Read the model definition and answer for the solid it produces. Units are mm, in the model's axes. Coordinates: 2 decimals unless noted, no trailing zeros. Order: outer loops, then holes, each group sorted by start corner. A loop starts at its lowest first (then second) coordinate and runs counter-clockwise, first axis right, second up.
```python
from build123d import *

# Parameters (mm, degrees)
SKETCH1_R           = 3
BOSS_EXTRUDE1_DEPTH = 114
CHAMFER1_SIZE       = 0.75
CHAMFER2_SIZE       = 0.75


with BuildPart() as part:
    # Sketch1 → Boss-Extrude1 (new body)
    with BuildSketch(Plane.XY):
        with Locations(Location((0, 0, 0), (0, 0, 180))):
            Circle(SKETCH1_R)
    extrude(amount=BOSS_EXTRUDE1_DEPTH)

    # Chamfer1
    chamfer1_edges = [part.edges().sort_by_distance(p)[0] for p in [
        (3, 0, 0),
    ]]
    chamfer(chamfer1_edges, length=CHAMFER1_SIZE)

    # Chamfer2
    chamfer2_edges = [part.edges().sort_by_distance(p)[0] for p in [
        (3, 0, 114),
    ]]
    chamfer(chamfer2_edges, length=CHAMFER2_SIZE)


solid = part.part
```
1) Straight lines are drawn through the part: line 1 (X direction, y = -0.2, z = 70); line 2 (Y direction, x = -1.1, z = 42); line 3 (Z direction, x = -1.2, y = 2.45). For each, find the intervals that lie inside material, in ascending order.
A:
line 1: x = -2.99 to 2.99
line 2: y = -2.79 to 2.79
line 3: z = 0.48 to 113.52
2) Flat-ended cylindrical pins translate along their axes: pin 1 Ø1 at (y, z) = (-1, 78) entering from +X; pin 2 Ø1 at (x, z) = (1, 41.5) entering from +Y; pin 3 Ø2 at (y, z) = (2.5, 52) entering from -X. Find the tip coordinate at first contact, or state that the pin passes through.
A:
pin 1: stops at x = 2.96
pin 2: stops at y = 2.96
pin 3: stops at x = -2.6
3) A cutting plane is placed at A-A, the plane z = 72.5. Determine the outline of the cut face in (x, y).
A:
outline: circle Ø6 at (0, 0)
